Input: part model. Units: mm. Frame: model coordinates. Face numbers are marked on the shaded views. Round coordinates to 2 decimals unless told otherwise and drop trailing zeros. Loops run counter-clockwise (first coordinate to the right, second up) from the corner with the lowest first, then second, coordinate; pieces in that order, holes last. Notation, with made-up numbers: (47.25, 65) - (57.25, 65) arc R5 ccw to (57.25, 70) - close; hole circle Ø3 at (-35.75, 50). An arc over 180 degrees is marked (long way). Write each question's results on one line, items separated by ' | '.
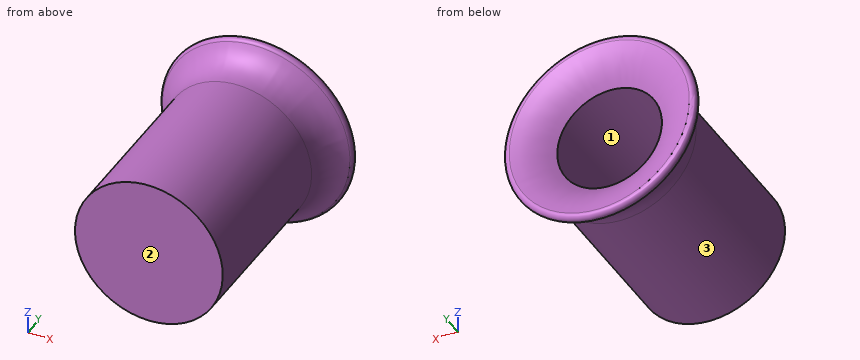
from build123d import *

# Parameters (mm, degrees)
SKETCH3_R          = 21.233227614
CUT_EXTRUDE1_DEPTH = 70


with BuildPart() as part:
    # Sketch1 → Revolve2 (revolve)
    with BuildSketch(Plane.XY, mode=Mode.PRIVATE) as revolve2_sk:
        with BuildLine():
            Line((0, 0), (30, 0))
            Line((30, 0), (30, 80))
            Line((30, 80), (8.888669742, 80))
            Line((8.888669742, 80), (8.766772386, 80))
            ThreePointArc((8.766772386, 80), (1.622655606, 85.063799106), (-6.577845512, 88.134995516))
            ThreePointArc((-6.577845512, 88.134995516), (-8.881517974, 86.949044637), (-8.081497092, 84.484627285))
            ThreePointArc((-8.081497092, 84.484627285), (-2.157248411, 78.299991195), (0, 70.011883734))
            Line((0, 70.011883734), (0, 0))
        make_face()
    revolve(revolve2_sk.sketch.rotate(Axis((30, 0, 0), (0, 1, 0)), 270), axis=Axis((30, 0, 0), (0, 1, 0)))

    # Sketch3 → Cut-Extrude1 (cut)
    with BuildSketch(Plane(origin=(0, 80, 0), x_dir=(1, 0, 0), z_dir=(0, 1, 0))):
        with Locations(Location((30, 0, 0), (0, 0, 270))):
            Circle(SKETCH3_R)
    extrude(amount=-CUT_EXTRUDE1_DEPTH, mode=Mode.SUBTRACT)


solid = part.part
1. Section query B-B, the plane x = 30. Output: boundary loops of the cut face in (y, z) (1 decimal), plus the area to 3 significant figures.
Answer:
outline: (0, -30) - (70, -30) arc R17 cw to (84.5, -38.1) arc R2 ccw to (88.1, -36.6) arc R34 ccw to (80, -21.2) - (10, -21.2) - (10, 21.2) - (80, 21.2) arc R34 ccw to (88.1, 36.6) arc R2 ccw to (84.5, 38.1) arc R17 cw to (70, 30) - (0, 30) - close | area: 2,000 mm^2
2. Section query A-A, the plane z = 0. Output: boundary loops of the cut face in (x, y) (1 decimal).
Answer:
outline: (-8.1, 84.5) arc R17 cw to (0, 70) - (0, 0) - (60, 0) - (60, 70) arc R17 cw to (68.1, 84.5) arc R2 ccw to (66.6, 88.1) arc R34 ccw to (51.2, 80) - (51.2, 10) - (8.8, 10) - (8.8, 80) arc R34 ccw to (-6.6, 88.1) arc R2 ccw to start
3. Section query C-C, the plane y = 20. Output: boundary loops of the cut face in (x, z), plus the area to 3 significant figures.
Answer:
outline: circle Ø60 at (30, 0); hole circle Ø42.47 at (30, 0) | area: 1,410 mm^2
4. Mould query, pull axis Z, two halves, no side actions, for the marked faces 1, 2 and 3. Classes: pulls with the +Z half, pulls with the -Z half, needs draft (parallel to the pull), parting line crosses it, or undercut.
Answer:
face 1: undercut | face 2: needs draft | face 3: parting line crosses it
5. Contact query for flat-ended pins moving along their axis: pin 1 (3 mm diameter, centred on x = 41, z = -2, fed in from +Y); pin 2 (10 mm diameter, centred on y = 18.5, z = -10, fed in from +X); pin 3 (5 mm diameter, centred on y = 27.5, z = 22, fed in from -X). Output: stop coordinate, or through.
Answer:
pin 1: y = 10 | pin 2: x = 59.58 | pin 3: x = 7.2
6. Line query: line 1 (X direction, y = 42.5, z = 0); line 2 (Y direction, x = 27, z = 19); line 3 (X direction, y = 35, z = -5). Output: solid intervals per line, ascending. Write a range as [from, to].
Answer:
line 1: [0, 8.77], [51.23, 60] | line 2: [0, 10] | line 3: [0.42, 9.36], [50.64, 59.58]
